The model under review builds one solid part; all positions refer to its coordinate system, in mm. A direction names the side the tool comes from. Give positions to 0.01 mm unless a question says otherwise; leave off trailing zeros. Order: outer loops, then holes, each group sorted by start corner. A loop starts at its lowest first (then second) coordinate and runs counter-clockwise, first axis right, second up. Notation, with made-up numbers: (75, 15) - (82, 15) arc R23 ccw to (82, 48) - close; hole circle Ø2 at (84, 37.5). An arc over 180 degrees is marked (long way). Put each result on its own line as item: value.
```python
from build123d import *

# Parameters (mm, degrees)
ESTRUSIONE_ESTRUSIONE1_START      = -11.2
SCHIZZO1_R                        = 3
ESTRUSIONE_ESTRUSIONE1_DEPTH      = 12
ESTRUSIONE_ESTRUSIONE1_DEPTH_BACK = 44
SMUSSO1_SIZE                      = 0.5
SCHIZZO4_R                        = 5
ESTRUSIONE_ESTRUSIONE2_DEPTH      = 6
TAGLIO_ESTRUSIONE1_DEPTH          = 2


with BuildPart() as part:
    # Schizzo1 → Estrusione-Estrusione1 (new body, two sides)
    with BuildSketch(Plane.XY.offset(ESTRUSIONE_ESTRUSIONE1_START)) as estrusione_estrusione1_sk:
        Circle(SCHIZZO1_R)
    extrude(amount=ESTRUSIONE_ESTRUSIONE1_DEPTH)
    extrude(estrusione_estrusione1_sk.sketch, amount=-ESTRUSIONE_ESTRUSIONE1_DEPTH_BACK)

    # Smusso1
    smusso1_edges = [part.edges().sort_by_distance(p)[0] for p in [
        (-3, 0, 0.8),
        (-3, 0, -55.2),
    ]]
    chamfer(smusso1_edges, length=SMUSSO1_SIZE)

    # Schizzo4 → Estrusione-Estrusione2 (add)
    with BuildSketch(Plane(origin=(0, 0, -55.2), x_dir=(-1, 0, 0), z_dir=(0, 0, -1))):
        Circle(SCHIZZO4_R)
    extrude(amount=-ESTRUSIONE_ESTRUSIONE2_DEPTH)

    # Schizzo6 → Taglio-Estrusione1 (cut)
    with BuildSketch(Plane(origin=(0, 0, -55.2), x_dir=(-1, 0, 0), z_dir=(0, 0, -1))):
        Polygon((1.5, 3), (-1.5, 3), (-3.232050808, 0), (-1.5, -3), (1.5, -3), (3.232050808, 0), align=None)
    extrude(amount=-TAGLIO_ESTRUSIONE1_DEPTH, mode=Mode.SUBTRACT)


solid = part.part
```
(1) Clearance check with flat-ended pins moving along their axes: pin 1 Ø3 at (y, z) = (-2, -14.5) entering from +X; pin 2 Ø1.5 at (x, y) = (1, 2) entering from -Z; pin 3 Ø2 at (x, z) = (0.5, -54) entering from -Y. State where each tip first meets the part, or that it passes through.
The answers:
pin 1: x = 2.96
pin 2: z = -53.2
pin 3: y = -5
(2) Take a section at A-A, the plane x = 0. Write out the cut boundary in (y, z), then the cut area to 3 significant figures.
The answers:
outline: (-5, -55.2) - (-3, -55.2) - (-3, -53.2) - (3, -53.2) - (3, -55.2) - (5, -55.2) - (5, -49.2) - (3, -49.2) - (3, 0.3) - (2.5, 0.8) - (-2.5, 0.8) - (-3, 0.3) - (-3, -49.2) - (-5, -49.2) - close
area: 348 mm^2
(3) Take a section at D-D, the plane y = -3.75. Write out the cut boundary in (x, z).
The answers:
outline: (-3.31, -55.2) - (3.31, -55.2) - (3.31, -49.2) - (-3.31, -49.2) - close
(4) For faces 4 (the flat face through (0, 0, -53.2)), 5 (the flat face through (-2.2, -2.2, -55.2)), list the 3-axis set-ups (+Z, -Z, +X, -X, +Y, -Y) from which the entire face can be reached by the end or side of a thin tool; tool diameter is ignored.
The answers:
face 4: -Z
face 5: -Z, +X, -X, +Y, -Y
(5) Take a section at B-B, the plane z = -50. Write out the cut boundary in (x, y), then the cut area to 3 significant figures.
The answers:
outline: circle Ø10 at (0, 0)
area: 78.5 mm^2
(6) The part is to be moulded in two halves that separate along X. For faces 1 (the cylindrical face through (-3, 0, -24)), 2 (the flat face through (0.1, -3.3, -49.2)), 3 (the flat face through (2.354, 1.521, -54.214)), say which applies: pulls with the +X half, pulls with the -X half, needs draft (parallel to the pull), parting line crosses it, or undercut.
The answers:
face 1: parting line crosses it
face 2: needs draft
face 3: undercut
(7) Take a section at C-C, the plane x = 4. Write out the cut boundary in (y, z), then the cut area to 3 significant figures.
The answers:
outline: (-3, -55.2) - (3, -55.2) - (3, -49.2) - (-3, -49.2) - close
area: 36.0 mm^2
(8) Wall thickness on L1, parallel to Z at x = 3.75, y = -1; L2, parallel to Z at x = 1, y = -1.75; L3, parallel to X at y = -2, z = -35: over which ranges is each line inside the solid? List them lowest first.
The answers:
L1: -55.2 to -49.2
L2: -53.2 to 0.8
L3: -2.24 to 2.24
